Read the model definition and answer for the solid it produces. Units are mm, in the model's axes. A direction names the side the tool comes from. Coordinates: 2 decimals unless noted, no trailing zeros. Write each loop counter-clockwise with the first axis right and the second up, starting at its lowest first coordinate (ties: lowest second). Pieces come first, ordered by that corner, then holes. Notation, with made-up numbers: (43, -29) - (81, -29) arc R31 ccw to (81, -4) - close; hole circle Ø1 at (68, 4.5). An arc over 180 degrees is marked (long way). Use a Markdown table: item, result.
from build123d import *

# Parameters (mm, degrees)
BOSS_EXTRU_1_DEPTH = 7.3
ESQUISSE2_R        = 2.25
BOSS_EXTRU_2_DEPTH = 5.2
CHANFREIN1_SIZE    = 1
CHANFREIN2_SIZE    = 1
CONG_1_R           = 1


with BuildPart() as part:
    # Esquisse1 → Boss.-Extru.1 (new body, symmetric)
    with BuildSketch(Plane.XY):
        with BuildLine():
            Line((-3.5, -1.936491673), (-3.5, -14.854191767))
            ThreePointArc((-3.5, -14.854191767), (-5.005210596, -19.361130861), (-8.916666667, -22.059031961))
            ThreePointArc((-8.916666667, -22.059031961), (-9.985168687, -23.710413809), (-8.5, -25))
            ThreePointArc((-8.5, -25), (-0.014718626, -21.485281374), (3.5, -13))
            Line((3.5, -13), (3.5, -1.936491673))
            ThreePointArc((3.5, -1.936491673), (4, 0), (3.5, 1.936491673))
            Line((3.5, 1.936491673), (3.5, 10))
            Line((3.5, 10), (-3.5, 10))
            Line((-3.5, 10), (-12.5, 10))
            Line((-12.5, 10), (-12.5, 5.2))
            Line((-12.5, 5.2), (-3.5, 5.2))
            Line((-3.5, 5.2), (-3.5, 1.936491673))
            ThreePointArc((-3.5, 1.936491673), (-4, 0), (-3.5, -1.936491673))
        make_face()
    extrude(amount=BOSS_EXTRU_1_DEPTH, both=True)

    # Esquisse2 → Boss.-Extru.2 (add)
    with BuildSketch(Plane.XY.offset(7.3)):
        Circle(ESQUISSE2_R)
    boss_extru_2 = extrude(amount=BOSS_EXTRU_2_DEPTH)

    # Chanfrein1
    chanfrein1_edges = [part.edges().sort_by_distance(p)[0] for p in [
        (-2.25, 0, 12.5),
    ]]
    chamfer(chanfrein1_edges, length=CHANFREIN1_SIZE)

    # Symétrie1: Boss.-Extru.2 across plane
    add(boss_extru_2.mirror(Plane.XY))

    # Chanfrein2
    chanfrein2_edges = [part.edges().sort_by_distance(p)[0] for p in [
        (-2.25, 0, -12.5),
    ]]
    chamfer(chanfrein2_edges, length=CHANFREIN2_SIZE)

    # Congé1
    cong_1_edges = [part.edges().sort_by_distance(p)[0] for p in [
        (3.5, -7.468245837, 7.3),
        (-5.005210596, -19.361130861, -7.3),
        (-3.5, -8.39534172, -7.3),
        (-4, 0, -7.3),
        (-3.5, 3.568245837, -7.3),
        (3.5, 5.968245837, -7.3),
        (4, 0, -7.3),
        (4, 0, 7.3),
        (3.5, -7.468245837, -7.3),
        (-0.014718626, -21.485281374, -7.3),
        (-9.985168687, -23.710413809, -7.3),
        (3.5, 5.968245837, 7.3),
        (-3.5, 3.568245837, 7.3),
        (-4, 0, 7.3),
        (-3.5, -8.39534172, 7.3),
        (-9.985168687, -23.710413809, 7.3),
        (-5.005210596, -19.361130861, 7.3),
        (-0.014718626, -21.485281374, 7.3),
    ]]
    fillet(cong_1_edges, radius=CONG_1_R)


solid = part.part
(1) Straight lines are drawn through the part: L1, parallel to Z at x = 2.5, y = 4.5; L2, parallel to X at y = -9.5, z = -5.5; L3, parallel to Y at x = -8.5, z = -4. For each, find the intervals that lie inside material, in ascending order.
Report:
| item | result |
|---|---|
| L1 | z = -7.3 to 7.3 |
| L2 | x = -3.5 to 3.5 |
| L3 | y = -25 to -21.93, 5.2 to 10 |
(2) The mould has two halves that part along Y. Classify faces 5 (the cylindrical face through (-0.29, 2.23, -9.37)), 6 (the flat face through (-2, -4, -7.3)), 7 (the cylindrical face through (-3.215, 3.404, 6.999)): pulls with the +Y half, pulls with the -Y half, needs draft (parallel to the pull), parting line crosses it, or undercut.
Report:
| item | result |
|---|---|
| face 5 | parting line crosses it |
| face 6 | needs draft |
| face 7 | undercut |
(3) A cutting plane is placed at C-C, the plane z = -8.75. Write down the section's boundary in (x, y).
Report:
| item | result |
|---|---|
| outline | circle Ø4.5 at (0, 0) |
(4) For faces 1 (the cylindrical face through (3.199, 5.888, -7.015)), 2 (the cylindrical face through (3.215, -7.25, 6.999)), 3 (the flat face through (3.5, 6, 0)), 4 (the flat face through (-3.5, -8, 0)), determine the directions among +Z, -Z, +X, -X, +Y, -Y from which every point of the face is accessible in a straight line to the end or side of a thin tool.
Report:
| item | result |
|---|---|
| face 1 | -Z, +X, +Y |
| face 2 | +Z, +X, -Y |
| face 3 | +Z, -Z, +X, +Y |
| face 4 | +Z, -Z, -X |
(5) A cutting plane is placed at B-B, the plane y = -4.5. Write down the section's boundary in (x, z), and give its area (3 significant figures).
Report:
| item | result |
|---|---|
| outline | (-3.5, -6.3) arc R1 ccw to (-2.5, -7.3) - (2.5, -7.3) arc R1 ccw to (3.5, -6.3) - (3.5, 6.3) arc R1 ccw to (2.5, 7.3) - (-2.5, 7.3) arc R1 ccw to (-3.5, 6.3) - close |
| area | 101 mm² |
(6) Each of these flat-tipped pins is pushed along its axis until it touches: P1, Ø6, axis at x = -10, y = 6, coming from the +Z side; P2, Ø3, axis at x = 2.5, z = 1.5, coming from the -Y side; P3, Ø3, axis at y = -4.5, z = -1.5, coming from the +X side. Where does it stop, or does it pass through?
Report:
| item | result |
|---|---|
| P1 | stops at z = 7.3 |
| P2 | stops at y = -20.33 |
| P3 | stops at x = 3.5 |
(7) A cutting plane is placed at A-A, the plane z = 3.25. Write down the section's boundary in (x, y).
Report:
| item | result |
|---|---|
| outline | (-12.5, 5.2) - (-3.5, 5.2) - (-3.5, 1.94) arc R4 ccw to (-3.5, -1.94) - (-3.5, -14.85) arc R7.5 cw to (-8.92, -22.06) arc R1.5 ccw to (-8.5, -25) arc R12 ccw to (3.5, -13) - (3.5, -1.94) arc R4 ccw to (3.5, 1.94) - (3.5, 10) - (-12.5, 10) - close |
